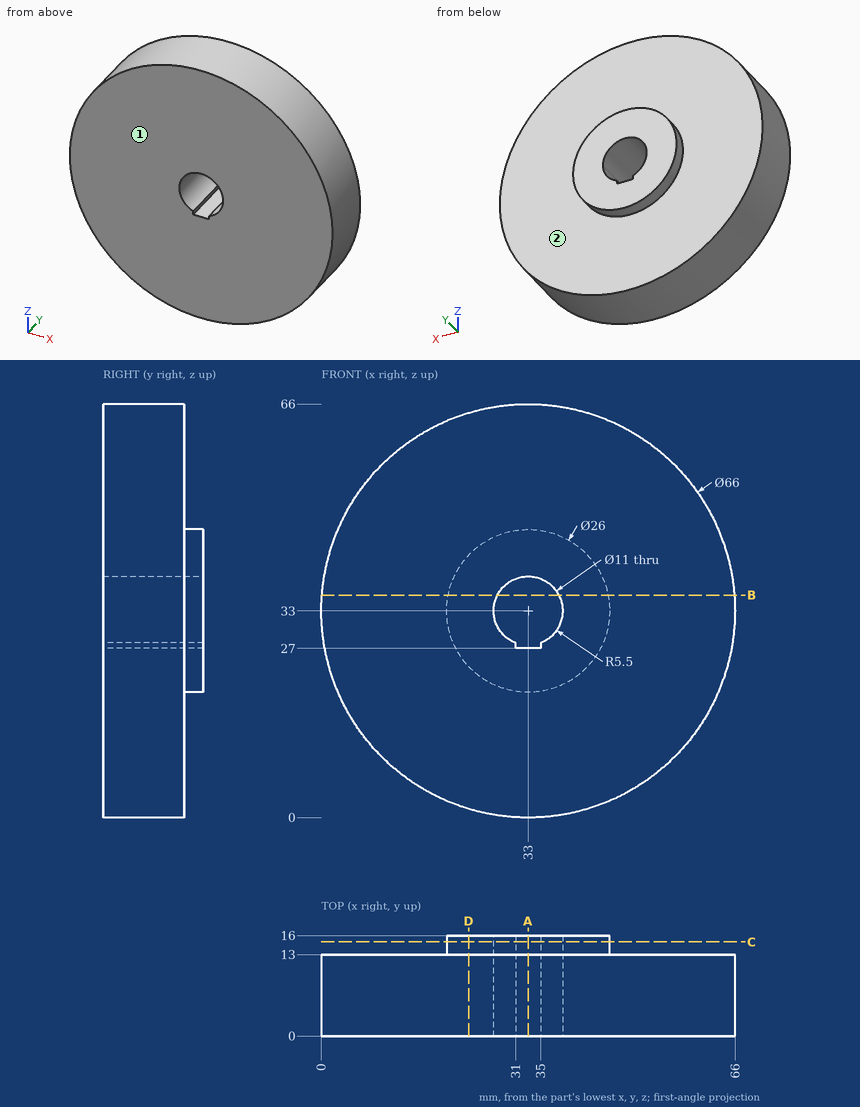
Source: three-view drawing plus pictorial views. Frame: mm from the lowest corner of the part. A direction names the side the tool comes from. Give positions to 0.01 mm unless a question says otherwise; leave off trailing zeros. Order: outer loops, then holes, each group sorted by start corner. A loop starts at its lowest first (then second) coordinate and runs counter-clockwise, first axis right, second up. Notation, with made-up numbers: (-9, 50.5) -> (19, 50.5) arc R15 cw to (19, 56.5) -> close; hole circle Ø6 at (-6, 65.25). An arc over 180 degrees is marked (long way). Use a Markdown table: item, result.
Q1. Section C-C (y = 15). Return the cut outline in (x, z), and give its area (3 significant figures).
A:
| item | result |
|---|---|
| outline | circle Ø26 at (33, 33); hole (31, 27) -> (35, 27) -> (35, 27.88) arc R5.5 ccw (long way) to (31, 27.88) -> close |
| area | 433 mm^2 |
Q2. First-contact query: P1, Ø1.2, axis at x = 32.5, y = 7, coming from the +Z side; P2, Ø3, axis at y = 13.5, z = 20, coming from the +X side; P3, Ø1.5, axis at y = 13, z = 54, coming from the -X side. Flat tips, straight axial feed; report the tip coordinate or a pass-through.
A:
| item | result |
|---|---|
| P1 | z = 66 |
| P2 | x = 63.9 |
| P3 | x = 6.94 |
Q3. Section A-A (x = 33). Return the cut outline in (y, z).
A:
| item | result |
|---|---|
| outline | (0, 0) -> (13, 0) -> (13, 20) -> (16, 20) -> (16, 27) -> (0, 27) -> close; (0, 38.5) -> (16, 38.5) -> (16, 46) -> (13, 46) -> (13, 66) -> (0, 66) -> close |
Q4. Material intervals for line 1 (Z direction, x = 33, y = 4.75); line 2 (X direction, y = 6, z = 33); line 3 (Y direction, x = 24.5, z = 6), sorted ascending. Write a range as [from, to].
A:
| item | result |
|---|---|
| line 1 | [0, 27], [38.5, 66] |
| line 2 | [0, 27.5], [38.5, 66] |
| line 3 | [0, 13] |
Q5. Access query for the marked faces 1 and 2. Directions: +Z, -Z, +X, -X, +Y, -Y. A direction counts if a zero-diameter tool reaches every point of the face in a straight line with its end or side. Return the directions, or none.
A:
| item | result |
|---|---|
| face 1 | +Z, -Z, +X, -X, -Y |
| face 2 | +Y |
Q6. Section D-D (x = 23.5). Return the cut outline in (y, z).
A:
| item | result |
|---|---|
| outline | (0, 1.4) -> (13, 1.4) -> (13, 24.13) -> (16, 24.13) -> (16, 41.87) -> (13, 41.87) -> (13, 64.6) -> (0, 64.6) -> close |
Q7. Section B-B (z = 35.5). Return the cut outline in (x, y), and give its area (3 significant figures).
A:
| item | result |
|---|---|
| outline | (0.09, 0) -> (28.1, 0) -> (28.1, 16) -> (20.24, 16) -> (20.24, 13) -> (0.09, 13) -> close; (37.9, 0) -> (65.91, 0) -> (65.91, 13) -> (45.76, 13) -> (45.76, 16) -> (37.9, 16) -> close |
| area | 775 mm^2 |
